Model file for the job. Use its own axes, mm. Coordinates: 2 decimals unless noted, no trailing zeros. Write each loop counter-clockwise with the first axis right and the second up, starting at its lowest first coordinate (ties: lowest second). Pieces come first, ordered by that corner, then holes. Notation, with made-up numbers: M 70.5,53.5 L 96.5,53.5 A13 ccw 96.5,70.5 Z; hole C 40,36.5 d10. An arc over 180 degrees is marked long. Use CSV: the item, a comma, the result in double quotes. Start each with the question number.
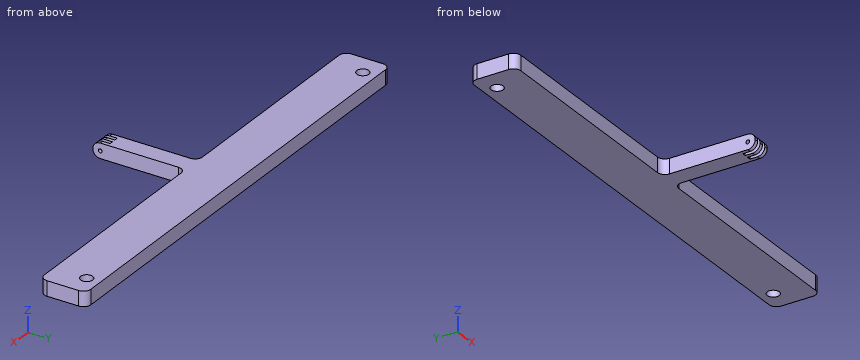
Autodesk Inventor part; units mm, degrees
ref_plane "YZ Plane" through (0, 0, 0) normal (1, 0, 0) x (0, 1, 0)
ref_plane "XZ Plane" through (0, 0, 0) normal (0, 1, 0) x (-1, 0, 0)
ref_plane "XY Plane" through (0, 0, 0) normal (0, 0, 1) x (1, 0, 0)
sketch "Sketch1" plane through (0, 0, 0) normal (0, 0, 1) x (1, 0, 0)
  line L0 (254, 0) -> (254, 25)
  line L1 (254, 25) -> (0, 25)
  line L2 (0, 25) -> (0, 0)
  line L3 (0, 25) -> (0, 21) construction
  line L4 (0, 21) -> (8.5, 21) construction
  line L5 (8.5, 21) -> (11.75, 21) construction
  line L6 (11.75, 21) -> (11.75, 17.75) construction
  circle A0 centre (11.75, 17.75) radius 3.25
  line L7 (254, 25) -> (254, 21) construction
  line L8 (254, 21) -> (245.5, 21) construction
  line L9 (245.5, 21) -> (245.5, 17.75) construction
  line L10 (245.5, 17.75) -> (242.25, 17.75) construction
  circle A1 centre (242.25, 17.75) radius 3.25
  line L11 (132, -50) -> (132, 0)
  line L12 (122, -50) -> (122, 0)
  line L13 (0, 0) -> (122, 0)
  line L14 (132, 0) -> (254, 0)
  line L15 (122, -50) -> (124, -50)
  line L16 (124, -50) -> (124, -42)
  line L17 (124, -42) -> (126, -42)
  line L18 (126, -42) -> (126, -50)
  line L19 (126, -50) -> (128, -50)
  line L20 (128, -50) -> (128, -42)
  line L21 (128, -42) -> (130, -42)
  line L22 (130, -42) -> (130, -50)
  line L23 (130, -50) -> (132, -50)
  dimension "d0" = 254
  dimension "d1" = 25
  dimension "d2" = 4
  dimension "d3" = 8.5
  dimension "d4" = 3.25
  dimension "d5" = 3.25
  dimension "d6" = 4
  dimension "d7" = 8.5
  dimension "d8" = 3.25
  dimension "d9" = 3.25
  dimension "d13" = 122
  dimension "d14" = 242.25
  dimension "d16" = 2
  dimension "d17" = 8
  dimension "d18" = 2
  dimension "d19" = 8
  dimension "d20" = 2
  dimension "d21" = 8
  dimension "d22" = 2
  dimension "d23" = 124
  dimension "d24" = 63
extrude "Extrusion1" add sketch "Sketch1" along normal blind 8
sketch "Sketch3" plane through (132, -50, 0) normal (1, 0, 0) x (0, 0, -1)
  line L0 (0, 0) -> (-8, 0)
  line L1 (0, 8) -> (-8, 8)
  line L2 (0, 0) -> (-8, 0) construction
  line L3 (-4, 0) -> (-4, 8) construction
  circle A0 centre (-4, 4) radius 1
  point P0 (0, 50)
  point P1 (-12, 0)
  point P2 (-12, 8)
  dimension "d39" = 2
extrude "Extrusion3" cut sketch "Sketch3" against normal blind 46.75
fillet "Fillet2" radius 4 6 edges at (127, -50, 8) (127, -50, 0) (123, -50, 0) (123, -50, 8) (131, -50, 0) (131, -50, 8)
fillet "Fillet4" radius 4 6 edges at (0, 25, 4) (0, 0, 4) (122, 0, 4) (132, 0, 4) (254, 0, 4) (254, 25, 4)
properties part number "WebcamBase"
1) Band-saw the part on C-C on z = 1.5. List the corners of the cut face in (x, y), then the cut area to 3 significant figures.
2) Drop flat-ended pins along their axis: P1, Ø4, axis at x = 196.5, z = 5, coming from the -Y side; P2, Ø2.5, axis at y = -21.5, z = 5.5, coming from the -X side; P3, Ø4, axis at y = -47, z = 3, coming from the +X side. Give the stop position or say it passes through.
3) Wall check: L1, parallel to Y at x = 127.45, z = 4; L2, parallel to Y at x = 242.25, z = 3.25; L3, parallel to Y at x = 211, z = 7.25. Give the ranges that are in metal, low to high. Write a range as [from, to].
4) Band-saw the part on D-D on y = -28. List the corners of the cut face in (x, z), then the cut area to 3 significant figures.
5) Band-saw the part on B-B on y = 17.75. List the corners of the cut face in (x, z), then the cut area to 3 significant figures.
6) Band-saw the part on A-A on x = 242.25. List the corners of the cut face in (y, z), then the cut area to 3 significant figures.
Findings below:
1,outline,"M 0,4 A4 ccw 4,0 L 118,0 A4 cw 122,-4 L 122,-49.12 L 124,-49.12 L 124,-42 L 126,-42 L 126,-49.12 L 128,-49.12 L 128,-42 L 130,-42 L 130,-49.12 L 132,-49.12 L 132,-4 A4 cw 136,0 L 250,0 A4 ccw 254,4 L 254,21 A4 ccw 250,25 L 4,25 A4 ccw 0,21 Z; hole C 11.75,17.75 d6.5; hole C 242.25,17.75 d6.5"
1,area,"6,740 mm2"
2,P1,"stops at y = 0"
2,P2,"stops at x = 122"
2,P3,"stops at x = 132"
3,L1,"y = [-50, -47], [-45, 25]"
3,L2,"y = [0, 14.5], [21, 25]"
3,L3,"y = [0, 25]"
4,outline,"M 122,0 L 132,0 L 132,8 L 122,8 Z"
4,area,"80.0 mm2"
5,outline,"M 0,0 L 8.5,0 L 8.5,8 L 0,8 Z; M 15,0 L 239,0 L 239,8 L 15,8 Z; M 245.5,0 L 254,0 L 254,8 L 245.5,8 Z"
5,area,"1,930 mm2"
6,outline,"M 0,0 L 14.5,0 L 14.5,8 L 0,8 Z; M 21,0 L 25,0 L 25,8 L 21,8 Z"
6,area,"148 mm2"
